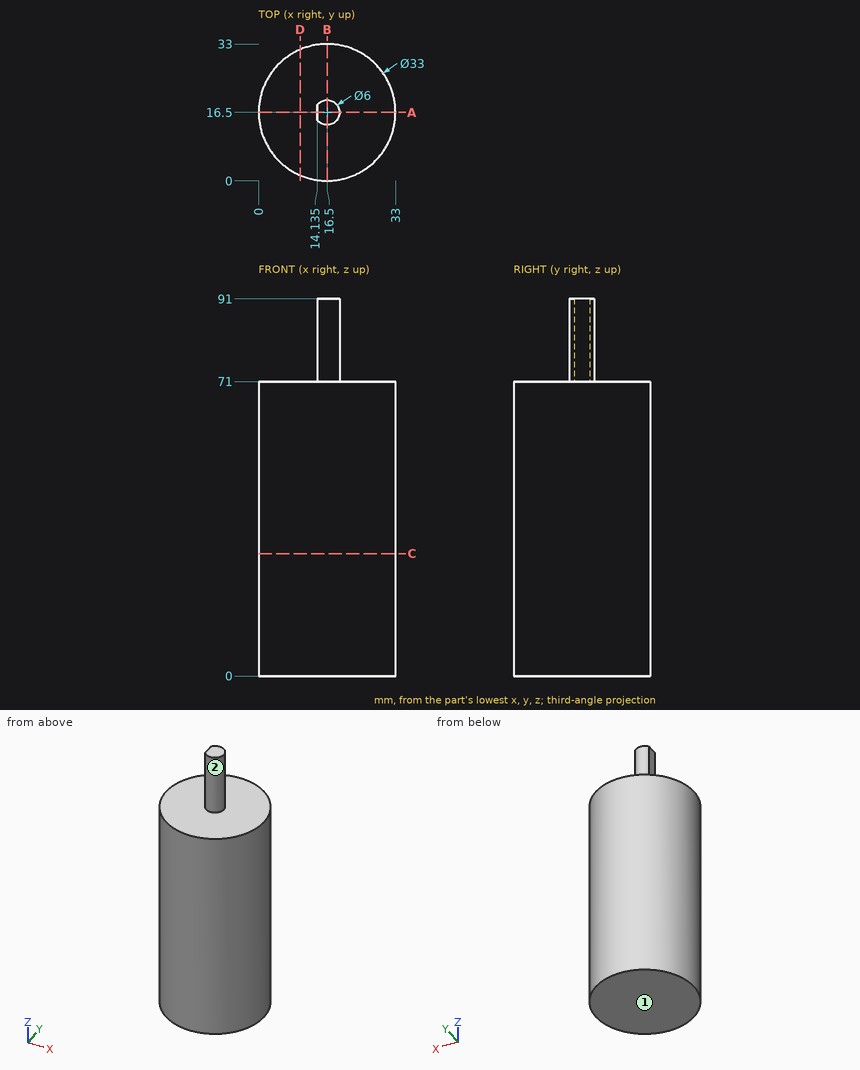
Drawing for the job (mm, zero at the part's lowest x, y, z). A direction names the side the tool comes from. Round coordinates to 2 decimals unless told otherwise and drop trailing zeros. Write each loop counter-clockwise with the first axis right and the second up, starting at its lowest first coordinate (ties: lowest second). Pieces come first, ordered by that corner, then holes. Notation, with made-up numbers: M 33.5,-19.75 L 91.5,-19.75 A14 ccw 91.5,5.25 Z; hole C 86.25,27 d10. An arc over 180 degrees is marked long. Answer as a JSON object with one key per item and string values. Group by question number.
(1) Cut at C-C (z = 29.5). Give the cut face in (x, y), and give its area (3 significant figures).
(2) Cut at D-D (x = 10). Give the cut face in (y, z) (1 decimal), and give its area (3 significant figures).
(3) Cut at B-B (x = 16.5). Give the cut face in (y, z).
(4) Drill centre lines: L1, parallel to Z at x = 8, y = 6; L2, parallel to Y at x = 17, z = 18.5; L3, parallel to X at y = 15.5, z = 69. Where is each one in solid material? Low to high.
(5) Cut at A-A (y = 16.5). Give the cut face in (x, z) (1 decimal).
(6) Which spindle directions (+Z, -Z, +X, -X, +Y, -Y) get a long thin tool onto all of the face, cutting with end or side? Do the marked faces 1 and 2. Say none if no direction does.
(7) Flat gauge pins, fed straight in: pin 1 (8 mm diameter, centred on x = 17, y = 7, fed in from -Z); pin 2 (3 mm diameter, centred on y = 16, z = 80.5, fed in from -X) (1 decimal); pin 3 (1.5 mm diameter, centred on x = 3.5, z = 33.5, fed in from +Y) (1 decimal); pin 4 (1 mm diameter, centred on y = 5, z = 18.5, fed in from +X). Where does each tip first touch, or does it go through?
Responses:
{
 "1": {"outline": "C 16.5,16.5 d33", "area": "855 mm2"},
 "2": {"outline": "M 1.3,0 L 31.7,0 L 31.7,71 L 1.3,71 Z", "area": "2,150 mm2"},
 "3": {"outline": "M 0,0 L 33,0 L 33,71 L 19.5,71 L 19.5,91 L 13.5,91 L 13.5,71 L 0,71 Z"},
 "4": {"L1": "z = 0 to 71", "L2": "y = 0.01 to 32.99", "L3": "x = 0.03 to 32.97"},
 "5": {"outline": "M 0,0 L 33,0 L 33,71 L 19.5,71 L 19.5,91 L 14.1,91 L 14.1,71 L 0,71 Z"},
 "6": {"face 1": "-Z, +X, -X, +Y, -Y", "face 2": "+Z"},
 "7": {"pin 1": "stops at z = 0", "pin 2": "stops at x = 14.1", "pin 3": "stops at y = 27.6", "pin 4": "stops at x = 28.8"}
}
